For this review, take the finished solid that the model builds, in its own axes (mm). Face numbers are marked on the shaded views. A direction names the side the tool comes from. Coordinates: 2 decimals unless noted, no trailing zeros. Loops run counter-clockwise (first coordinate to the right, second up) from the corner with the lowest first, then second, coordinate; pieces in that order, holes last. Notation, with made-up numbers: M -29,60.25 L -18,60.25 A28 ccw -18,92.25 Z; hole C 53.25,79 d7. An arc over 180 degrees is marked long. Write item = value, one per line.
from build123d import *

# Parameters (mm, degrees)
F2_R     = 21
F3_DEPTH = 14
F4_T     = -3
F6_D     = 4
F7_D     = 16


with BuildPart() as f3:
    # F2 (on Top) → F3 (new body)
    with BuildSketch(Plane.XY):
        Circle(F2_R)
    extrude(amount=F3_DEPTH)

    # F4
    f4_openings = [f3.faces().sort_by_distance(p)[0] for p in [
        (0, 0, 14),
    ]]
    offset(amount=F4_T, openings=f4_openings)

    # F6 (through all)
    with Locations(Plane(origin=(0, 0, 0), x_dir=(1, 0, 0), z_dir=(0, 0, -1))):
        with Locations((-12.5, 0), (0, 12.5), (12.5, 0), (0, -12.5)):
            Hole(F6_D / 2)

    # F7 (through all)
    with Locations(Plane(origin=(0, 0, 0), x_dir=(1, 0, 0), z_dir=(0, 0, -1))):
        with Locations((0, 0)):
            Hole(F7_D / 2)


solid = f3.part
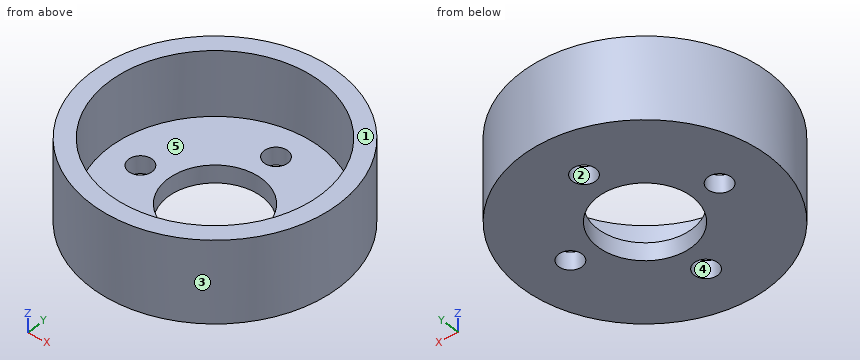
Q1. Machinability: for the marked faces 4 and 5, which of the approach directions +Z, -Z, +X, -X, +Y, -Y give a long, thin tool a straight path to every point of the face, cutting with its end or side? Answer none if there is none.
Solved:
face_4 = +Z, -Z
face_5 = +Z
Q2. For pin 1 Ø6 at (y, z) = (-5, 5) entering from +X; pin 2 Ø1 at (y, z) = (10.5, 7) entering from -X; pin 3 Ø4 at (y, z) = (-9.5, 10) entering from -X; pin 4 Ø3.5 at (x, y) = (-12.5, 0) entering from +Z, all flat-tipped, find the tip position at first contact; note any pin that passes through.
Solved:
pin_1 = 20.9
pin_2 = -18.47
pin_3 = -19.62
pin_4 = through
Q3. For line 1 along Y through (x, z) = (0, 1.65); line 2 along Y through (x, z) = (0.5, 12); line 3 along Z through (x, y) = (7, 12), list the stretches that pass through material, from the lowest coordinate up.
Solved:
line_1 = -21 to -14.5, -10.5 to -8, 8 to 10.5, 14.5 to 21
line_2 = -20.99 to -17.99, 17.99 to 20.99
line_3 = 0 to 3
Q4. Draft analysis for pull direction X (two halves, no side actions). For the marked faces 1, 2 and 3, state which applies: +X half, -X half, draft (parallel to the pull), parting line (faces both ways), or undercut.
Solved:
face_1 = draft
face_2 = undercut
face_3 = parting line
Q5. Add section C-C (x = -6.5). Write out the cut boundary in (y, z), and give its area (3 significant figures).
Solved:
outline = M -19.97,0 L -4.66,0 L -4.66,3 L -16.79,3 L -16.79,14 L -19.97,14 Z; M 4.66,0 L 19.97,0 L 19.97,14 L 16.79,14 L 16.79,3 L 4.66,3 Z
area = 162 mm²
Q6. Add section D-D (y = 11). Write out the cut boundary in (x, z), and give its area (3 significant figures).
Solved:
outline = M -17.89,0 L -1.32,0 L -1.32,3 L -14.25,3 L -14.25,14 L -17.89,14 Z; M 1.32,0 L 17.89,0 L 17.89,14 L 14.25,14 L 14.25,3 L 1.32,3 Z
area = 179 mm²
Q7. Add section A-A (x = 0). Write out the cut boundary in (y, z), and give its area (3 significant figures).
Solved:
outline = M -21,0 L -14.5,0 L -14.5,3 L -18,3 L -18,14 L -21,14 Z; M -10.5,0 L -8,0 L -8,3 L -10.5,3 Z; M 8,0 L 10.5,0 L 10.5,3 L 8,3 Z; M 14.5,0 L 21,0 L 21,14 L 18,14 L 18,3 L 14.5,3 Z
area = 120 mm²
